The listing builds one solid part. Answer for the finished solid, in the listing's coordinates (mm). A direction names the side the tool comes from. Give positions to 0.01 mm unless a question says otherwise; leave off trailing zeros. Order: outer loops, then holes, each group sorted by start corner. A loop starts at its lowest first (then second) coordinate and runs counter-clockwise, first axis right, second up. Notation, with made-up numbers: (1.25, 25.25) -> (26.25, 25.25) arc R14 cw to (26.25, 51.25) -> close; hole circle Ø3 at (38, 23.25). An arc over 180 degrees is marked (long way). Answer as a JSON object with one key per item and string values. Group by question number.
```python
from build123d import *

# Parameters (mm, degrees)
SKETCH_1_W             = 372
SKETCH_1_H             = 115
SM_BASE_FLANGE_1_DEPTH = 1
SKETCH_6_W             = 342
SKETCH_6_H             = 95
CUT_EXTRUDE_1_DEPTH    = 10
CUT_EXTRUDE_2_DEPTH    = 10
PATTERN_LINEAR_1_COUNT = 4
PATTERN_LINEAR_1_PITCH = 95
OTHER_START            = -38
OTHER_1_DEPTH          = 76
OTHER_1_2_DEPTH        = 0.5
OTHER_START_2          = 37.5
OTHER_1_3_DEPTH        = 0.5
OTHER_START_3          = -37.5
OTHER_1_4_DEPTH        = 75
SKETCH_15_W            = 11.7634
SKETCH_15_H            = 29
CUT_EXTRUDE_3_DEPTH    = 10
FILLET_1_R             = 5
FILLET_2_R             = 1
FILLET_1_OF_MIRROR_1_R = 5
FILLET_2_OF_MIRROR_1_R = 1


# Read off the part's stored shape, not the designer's step: 斜接法兰1
# Sheet-metal steps are written as plain solids
with BuildPart() as part:
    # Sketch 1 → 基体-法兰1 (new body)
    with BuildSketch(Plane.XY):
        Rectangle(SKETCH_1_W, SKETCH_1_H)
    extrude(amount=-SM_BASE_FLANGE_1_DEPTH)

    # 草图6 → 切除-拉伸1 (cut)
    with BuildSketch(Plane.XY):
        Rectangle(SKETCH_6_W, SKETCH_6_H)
    extrude(amount=-CUT_EXTRUDE_1_DEPTH, mode=Mode.SUBTRACT)

    # 草图7 → 切除-拉伸2 (cut)
    with BuildSketch(Plane.XY):
        with BuildLine():
            Line((-176, 55.5), (-116, 55.5))
            ThreePointArc((-116, 55.5), (-113, 52.5), (-116, 49.5))
            Line((-116, 49.5), (-176, 49.5))
            ThreePointArc((-176, 49.5), (-179, 52.5), (-176, 55.5))
        make_face()
        with BuildLine():
            Line((-176, -55.5), (-116, -55.5))
            ThreePointArc((-116, -55.5), (-113, -52.5), (-116, -49.5))
            Line((-116, -49.5), (-176, -49.5))
            ThreePointArc((-176, -49.5), (-179, -52.5), (-176, -55.5))
        make_face()
    cut_extrude_2 = extrude(amount=-CUT_EXTRUDE_2_DEPTH, mode=Mode.SUBTRACT)

    # 阵列(线性)1: 切除-拉伸2 ×4
    with Locations(*[(i * PATTERN_LINEAR_1_PITCH, 0, 0) for i in range(1, PATTERN_LINEAR_1_COUNT)]):
        add(cut_extrude_2, mode=Mode.SUBTRACT)

    # Other 1 outline → Other 1 (cut)
    with BuildSketch(Plane(origin=(0, 0, 0), x_dir=(1, 0, 0), z_dir=(0, 1, 0)).offset(OTHER_START)):
        with BuildLine():
            Line((186, 1), (185.83604109, 1))
            ThreePointArc((185.83604109, 1), (185.195226164, 0.271171885), (184.2634, 0))
            Line((184.2634, 0), (186, 0))
            Line((186, 0), (186, 1))
        make_face()
    other_1 = extrude(amount=OTHER_1_DEPTH, mode=Mode.SUBTRACT)

    # Other 1 2 outline → Other 1 2 (cut)
    with BuildSketch(Plane(origin=(0, 0, 0), x_dir=(1, 0, 0), z_dir=(0, 1, 0)).offset(OTHER_START)):
        with BuildLine():
            ThreePointArc((184.2634, 0), (185.195226164, 0.271171885), (185.83604109, 1))
            Line((185.83604109, 1), (183.7634, 1))
            Line((183.7634, 1), (183.7634, 0))
            Line((183.7634, 0), (184.2634, 0))
        make_face()
    other_1_2 = extrude(amount=OTHER_1_2_DEPTH, mode=Mode.SUBTRACT)

    # Other 1 3 outline → Other 1 3 (cut)
    with BuildSketch(Plane(origin=(0, 0, 0), x_dir=(1, 0, 0), z_dir=(0, 1, 0)).offset(OTHER_START_2)):
        with BuildLine():
            ThreePointArc((184.2634, 0), (185.195226164, 0.271171885), (185.83604109, 1))
            Line((185.83604109, 1), (183.7634, 1))
            Line((183.7634, 1), (183.7634, 0))
            Line((183.7634, 0), (184.2634, 0))
        make_face()
    other_1_3 = extrude(amount=OTHER_1_3_DEPTH, mode=Mode.SUBTRACT)

    # Other 1 4 outline → Other 1 4 (add)
    with BuildSketch(Plane(origin=(0, 0, 0), x_dir=(1, 0, 0), z_dir=(0, 1, 0)).offset(OTHER_START_3)):
        with BuildLine():
            Line((186, 1.7366), (186, 5.2634))
            ThreePointArc((186, 5.2634), (186.215745145, 5.784254855), (186.7366, 6))
            Line((186.7366, 6), (198.5, 6))
            Line((198.5, 6), (198.5, 7))
            Line((198.5, 7), (186.7366, 7))
            ThreePointArc((186.7366, 7), (185.508638364, 6.491361636), (185, 5.2634))
            Line((185, 5.2634), (185, 1.7366))
            ThreePointArc((185, 1.7366), (184.784254855, 1.215745145), (184.2634, 1))
            Line((184.2634, 1), (185.83604109, 1))
            ThreePointArc((185.83604109, 1), (185.958514757, 1.359286442), (186, 1.7366))
        make_face()
    other_1_4 = extrude(amount=OTHER_1_4_DEPTH)

    # 草图15 → 切除-拉伸3 (cut)
    with BuildSketch(Plane(origin=(0, 0, -7), x_dir=(-1, 0, 0), z_dir=(0, 0, -1))):
        with Locations((-192.6183, 0)):
            Rectangle(SKETCH_15_W, SKETCH_15_H)
    cut_extrude_3 = extrude(amount=-CUT_EXTRUDE_3_DEPTH, mode=Mode.SUBTRACT)

    # 圆角1
    fillet_1_edges = [part.edges().sort_by_distance(p)[0] for p in [
        (198.5, -37.5, -6.5),
        (198.5, 37.5, -6.5),
        (198.5, -14.5, -6.5),
        (198.5, 14.5, -6.5),
    ]]
    fillet(fillet_1_edges, radius=FILLET_1_R)

    # 圆角2
    fillet_2_edges = [part.edges().sort_by_distance(p)[0] for p in [
        (184.0134, -37.5, 0),
        (184.0134, 37.5, 0),
        (186, -37.5, -3.5),
        (186, 37.5, -3.5),
        (186.215745145, 37.5, -5.784254855),
        (186.215745145, -37.5, -5.784254855),
        (190.1183, -37.5, -6),
        (185.195226164, -37.5, -0.271171885),
        (185.195226164, 37.5, -0.271171885),
        (190.1183, -14.5, -6),
        (198.5, 26, -6),
        (190.1183, 14.5, -6),
        (190.1183, 37.5, -6),
        (197.035533906, 36.035533906, -6),
        (197.035533906, 15.964466094, -6),
        (198.5, -26, -6),
        (197.035533906, -15.964466094, -6),
        (197.035533906, -36.035533906, -6),
    ]]
    fillet(fillet_2_edges, radius=FILLET_2_R - 0.0001)  # a hair under: the kernel refuses the full size

    # 镜向1: Other 1, Other 1 2, Other 1 3, Other 1 4, 切除-拉伸3 across plane
    add(other_1.mirror(Plane(origin=(0, 0, 0), x_dir=(0, 0, 1), z_dir=(1, 0, 0))), mode=Mode.SUBTRACT)
    add(other_1_2.mirror(Plane(origin=(0, 0, 0), x_dir=(0, 0, 1), z_dir=(1, 0, 0))), mode=Mode.SUBTRACT)
    add(other_1_3.mirror(Plane(origin=(0, 0, 0), x_dir=(0, 0, 1), z_dir=(1, 0, 0))), mode=Mode.SUBTRACT)
    add(other_1_4.mirror(Plane(origin=(0, 0, 0), x_dir=(0, 0, 1), z_dir=(1, 0, 0))))
    add(cut_extrude_3.mirror(Plane(origin=(0, 0, 0), x_dir=(0, 0, 1), z_dir=(1, 0, 0))), mode=Mode.SUBTRACT)

    # 圆角1 of 镜向1
    fillet_1_of_mirror_1_edges = [part.edges().sort_by_distance(p)[0] for p in [
        (-198.5, -37.5, -6.5),
        (-198.5, 37.5, -6.5),
        (-198.5, -14.5, -6.5),
        (-198.5, 14.5, -6.5),
    ]]
    fillet(fillet_1_of_mirror_1_edges, radius=FILLET_1_OF_MIRROR_1_R)

    # 圆角2 of 镜向1
    fillet_2_of_mirror_1_edges = [part.edges().sort_by_distance(p)[0] for p in [
        (-184.0134, -37.5, 0),
        (-184.0134, 37.5, 0),
        (-186, -37.5, -3.5),
        (-186, 37.5, -3.5),
        (-186.215745145, 37.5, -5.784254855),
        (-186.215745145, -37.5, -5.784254855),
        (-190.1183, -37.5, -6),
        (-185.195226164, -37.5, -0.271171885),
        (-185.195226164, 37.5, -0.271171885),
        (-190.1183, -14.5, -6),
        (-198.5, 26, -6),
        (-190.1183, 14.5, -6),
        (-190.1183, 37.5, -6),
        (-197.035533906, 36.035533906, -6),
        (-197.035533906, 15.964466094, -6),
        (-198.5, -26, -6),
        (-197.035533906, -15.964466094, -6),
        (-197.035533906, -36.035533906, -6),
    ]]
    fillet(fillet_2_of_mirror_1_edges, radius=FILLET_2_OF_MIRROR_1_R - 0.0001)  # a hair under: the kernel refuses the full size


solid = part.part
```
(1) A cutting plane is placed at A-A (x = 36). Determine the outline of the cut face in (y, z), and give its area (3 significant figures).
(2) A cutting plane is placed at B-B (y = 9.5). Determine the outline of the cut face in (x, z), and give its area (3 significant figures).
(3) A cutting plane is placed at D-D (x = 96). Determine the outline of the cut face in (y, z).
(4) Which of the six approach directions +Z, -Z, +X, -X, +Y, -Y give full straight-line access (tool end or side, diameter ignored) to faces 1 (the flat face through (-192, -26, -6)), 2 (the flat face through (193, -26, -7)), 3 (the flat face through (192, -26, -6))?
(5) Find the intervals of material crossed by line 1 along X through (y, z) = (-13, -1.5); line 2 along Y through (x, z) = (6, -0.5); line 3 along X through (y, z) = (-4, -6.25), in increasing order. Write a range as [from, to].
(6) Flat-ended cylindrical pins translate along their axes: pin 1 Ø1.5 at (y, z) = (12.5, -4.5) entering from +X; pin 2 Ø8.5 at (x, y) = (189.5, 28.5) entering from +Z; pin 3 Ø3 at (x, z) = (186.5, -3) entering from -Y; pin 4 Ø3 at (x, z) = (-188.5, -2.5) entering from +Y. Find the tip coordinate at first contact, or state that the pin passes through.
Check sheet entries:
{
 "1": {"outline": "(-57.5, -1) -> (-55.5, -1) -> (-55.5, 0) -> (-57.5, 0) -> close; (-49.5, -1) -> (-47.5, -1) -> (-47.5, 0) -> (-49.5, 0) -> close; (47.5, -1) -> (49.5, -1) -> (49.5, 0) -> (47.5, 0) -> close; (55.5, -1) -> (57.5, -1) -> (57.5, 0) -> (55.5, 0) -> close", "area": "8.00 mm2"},
 "2": {"outline": "(-186.74, -7) arc R1.74 ccw to (-185, -5.26) -> (-185, -1.74) arc R0.74 cw to (-184.26, -1) -> (-171, -1) -> (-171, 0) -> (-184.26, 0) arc R1.74 ccw to (-186, -1.74) -> (-186, -5.26) arc R0.74 cw to (-186.74, -6) -> close; (171, -1) -> (184.26, -1) arc R0.74 cw to (185, -1.74) -> (185, -5.26) arc R1.74 ccw to (186.74, -7) -> (186.74, -6) arc R0.74 cw to (186, -5.26) -> (186, -1.74) arc R1.74 ccw to (184.26, 0) -> (171, 0) -> close", "area": "41.4 mm2"},
 "3": {"outline": "(-57.5, -1) -> (-47.5, -1) -> (-47.5, 0) -> (-57.5, 0) -> close; (47.5, -1) -> (57.5, -1) -> (57.5, 0) -> (47.5, 0) -> close"},
 "4": {"face 1": "+Z, -X, +Y, -Y", "face 2": "-Z, +X, -X, +Y, -Y", "face 3": "+Z, +X, +Y, -Y"},
 "5": {"line 1": "x = [-185.98, -184.96], [184.96, 185.98]", "line 2": "y = [-57.5, -47.5], [47.5, 57.5]", "line 3": "x = [-186.74, -185.31], [185.31, 186.74]"},
 "6": {"pin 1": "stops at x = 186", "pin 2": "stops at z = -0.31", "pin 3": "stops at y = -37.5", "pin 4": "passes through"}
}
